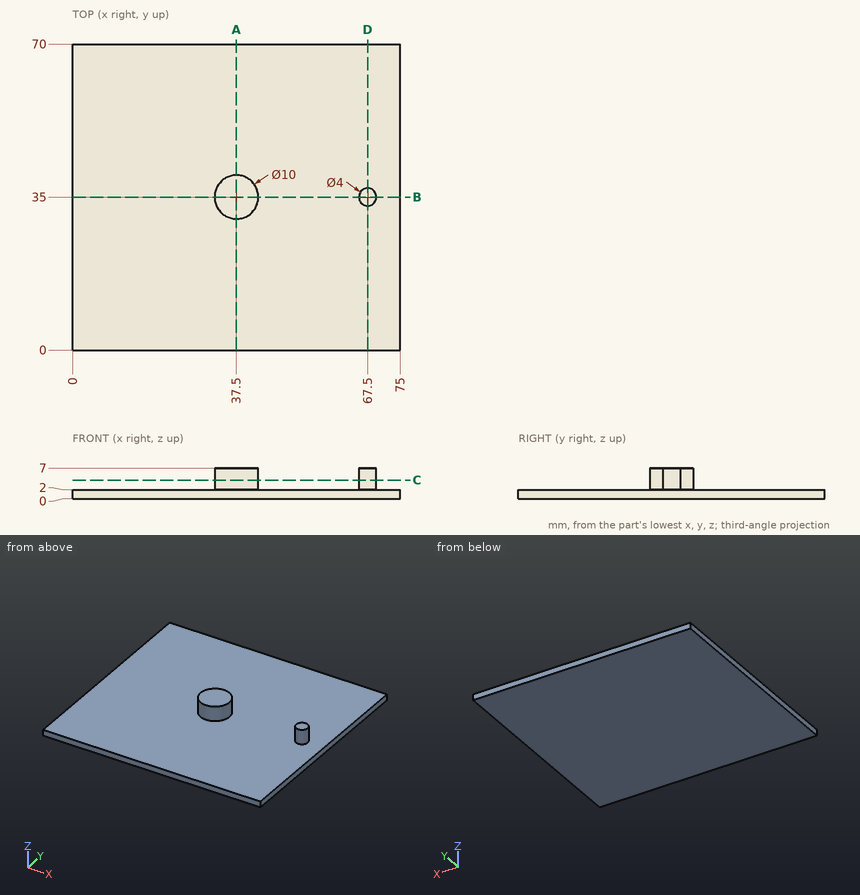
Could you check a few things on this drawing? It's one solid part, dimensions in mm from its lowest x, y, z. Give positions to 0.01 mm unless a question says otherwise; leave off trailing zeros. Write each loop counter-clockwise with the first axis right and the second up, starting at its lowest first coordinate (ties: lowest second). Pieces come first, ordered by that corner, then holes. Notation, with made-up numbers: (31.5, 24.5) -> (63.5, 24.5) arc R18 ccw to (63.5, 30.5) -> close; hole circle Ø3 at (20.5, 69.5). An arc over 180 degrees is marked (long way). Write item = value, one per line.
(1) Suppose I cut it at A-A on x = 37.5. Write out the boundary of the cut face in (y, z), then the cut area to 3 significant figures.
Worked out:
outline = (0, 0) -> (70, 0) -> (70, 2) -> (40, 2) -> (40, 7) -> (30, 7) -> (30, 2) -> (0, 2) -> close
area = 190 mm^2
(2) Suppose I cut it at B-B on y = 35. Write out the boundary of the cut face in (x, z).
Worked out:
outline = (0, 0) -> (75, 0) -> (75, 2) -> (69.5, 2) -> (69.5, 7) -> (65.5, 7) -> (65.5, 2) -> (42.5, 2) -> (42.5, 7) -> (32.5, 7) -> (32.5, 2) -> (0, 2) -> close
(3) I'm going to push flat-ended pins straight in: P1, Ø3, axis at x = 22.5, y = 31.5, coming from the +Z side; P2, Ø3, axis at x = 37, z = 5.5, coming from the +Y side. Where does each tip first touch, or does it pass through?
Worked out:
P1 = 2
P2 = 40
(4) I need wall thicknesses on probe 1 along Z at (x, y) = (16, 25); probe 2 along X at (y, z) = (35.5, 6); probe 3 along Y at (x, z) = (33, 4). Which ranges of each line are inside material? Lowest first, please. Write a range as from..to.
Worked out:
probe_1 = 0..2
probe_2 = 32.53..42.47, 65.56..69.44
probe_3 = 32.82..37.18
(5) Suppose I cut it at D-D on x = 67.5. Write out the boundary of the cut face in (y, z).
Worked out:
outline = (0, 0) -> (70, 0) -> (70, 2) -> (37, 2) -> (37, 7) -> (33, 7) -> (33, 2) -> (0, 2) -> close
(6) Suppose I cut it at C-C on z = 4.25. Write out the boundary of the cut face in (x, y).
Worked out:
outline = circle Ø10 at (37.5, 35); circle Ø4 at (67.5, 35)
